Here's how the part is built. I have some questions about the finished solid (model axes, mm). A direction names the side the tool comes from. Round coordinates to 2 decimals unless told otherwise and drop trailing zeros. Write each loop counter-clockwise with the first axis right and the second up, starting at its lowest first coordinate (ties: lowest second). Pieces come first, ordered by that corner, then holes. Notation, with made-up numbers: (-15.5, -12) -> (-9.5, -12) arc R23 ccw to (-9.5, 15) -> close; hole circle Ø10 at (80, 14.25). An arc over 180 degrees is marked (long way). Put each result on its own line as item: value. Start each with the question number.
1. For pin 1 (5 mm diameter, centred on y = 6.5, z = 2199, fed in from +X); pin 2 (10 mm diameter, centred on y = 32, z = 901.5, fed in from -X); pin 3 (5 mm diameter, centred on x = 27, y = -12, fed in from -Z), each with a flat end and sliding along its axis, tell me the tip position at first contact or that it passes through.
2. I need wall thicknesses on probe 1 along Y at (x, z) = (33.5, 731); probe 2 along Y at (x, z) = (-6.5, 903.5); probe 3 along X at (y, z) = (20, 2338). Which ranges of each line are inside material? Lowest first, please. Write a range as from..to.
3. Which directions (+Z, -Z, +X, -X, +Y, -Y) give clear straight access to the entire face, cutting with the end or side of a thin tool? Please do faces 1 (the face through (-62.264, -36.012, 1355.242)), 2 (the face through (67, -37, 2743.2)), 3 (the face through (62.264, 36.012, 1355.242)).
4. Suppose I cut it at A-A (z = 2237.5). Please give me the cut outline in (x, y), then the cut area to 3 significant figures.
```python
from build123d import *

# Parameters (mm, degrees)
F1_DEPTH     = 2540
F3_DEPTH     = 203.2
F4_R         = 76.1921609871
F5_DEPTH     = 101.6
F6_SIZE2     = 203.2
F6_SIZE      = 71.882
F7_T1_DEPTH  = 494.4083201135
F7_T3_DEPTH  = 494.4083201135
F7_T5_DEPTH  = 494.4083201135
F7_T7_DEPTH  = 494.4083201135
F7_T9_DEPTH  = 494.4083201135
F7_T11_DEPTH = 494.4083201135


# Not quite as in the source:
# - a fillet or chamfer that OpenCascade refuses, or shapes differently, is made with other operations: its cross-section is extruded or revolved along the edge and cut away or added


with BuildPart() as f1:
    # F0 (on Top) → F1 (new body)
    with BuildSketch(Plane.XY):
        Polygon((42.1619373396, -71.5559341018), (83.0502253935, 0.735341758), (40.8882880539, 72.2912758598), (-42.1619373396, 71.5559341018), (-83.0502253935, -0.735341758), (-40.8882880539, -72.2912758598), align=None)
    extrude(amount=F1_DEPTH)

    # F2 (on face) → F3 (join)
    with BuildSketch(Plane.XY.offset(2540)):
        with BuildLine():
            ThreePointArc((-40.8882880539, -72.2912758598), (0.735341758, -83.0502253935), (42.1619373396, -71.5559341018))
            Line((42.1619373396, -71.5559341018), (-40.8882880539, -72.2912758598))
        make_face()
        with BuildLine():
            ThreePointArc((-83.0502253935, -0.735341758), (-71.5559341018, -42.1619373396), (-40.8882880539, -72.2912758598))
            Line((-40.8882880539, -72.2912758598), (-83.0502253935, -0.735341758))
        make_face()
        with BuildLine():
            Line((-83.0502253935, -0.735341758), (-42.1619373396, 71.5559341018))
            ThreePointArc((-42.1619373396, 71.5559341018), (-72.2912758598, 40.8882880539), (-83.0502253935, -0.735341758))
        make_face()
        Polygon((42.1619373396, -71.5559341018), (83.0502253935, 0.735341758), (40.8882880539, 72.2912758598), (-42.1619373396, 71.5559341018), (-83.0502253935, -0.735341758), (-40.8882880539, -72.2912758598), align=None)
        with BuildLine():
            ThreePointArc((42.1619373396, -71.5559341018), (72.1095566371, -41.2079180135), (83.0534807543, 0))
            ThreePointArc((83.0534807543, 0), (83.0526669101, 0.3676744818), (83.0502253935, 0.735341758))
            Line((83.0502253935, 0.735341758), (42.1619373396, -71.5559341018))
        make_face()
        with BuildLine():
            Line((40.8882880539, 72.2912758598), (83.0502253935, 0.735341758))
            ThreePointArc((83.0502253935, 0.735341758), (71.5559341018, 42.1619373396), (40.8882880539, 72.2912758598))
        make_face()
        with BuildLine():
            Line((-42.1619373396, 71.5559341018), (40.8882880539, 72.2912758598))
            ThreePointArc((40.8882880539, 72.2912758598), (-0.735341758, 83.0502253935), (-42.1619373396, 71.5559341018))
        make_face()
    extrude(amount=F3_DEPTH)

    # F4 (on face) → F5 (join)
    with BuildSketch(Plane.XY.offset(2743.2)):
        Circle(F4_R)
    extrude(amount=F5_DEPTH)

    # F6
    f6_edges = [f1.edges().sort_by_distance(p)[0] for p in [
        (62.606081, -35.410296, 0),
        (61.969257, 36.513309, 0),
        (-0.636825, 71.923605, 0),
        (-62.606081, 35.410296, 0),
        (-61.969257, -36.513309, 0),
        (0.636825, -71.923605, 0),
    ]]
    f6_side = f1.faces().sort_by_distance((0, 0, 0))[0]
    chamfer(f6_edges, length=F6_SIZE, length2=F6_SIZE2, reference=f6_side)

    # F7: fillet of radius 76.2 on 6 edges, made by hand

    # F7_s2 → F7_t1 (cut)
    with BuildSketch(Plane(origin=(-18.9514614698, -33.5065465998, -94.2401135792), x_dir=(-0.8704183762, 0.4923127566, 0), z_dir=(0.1861654151, 0.329144017, 0.9257465389))):
        with BuildLine():
            ThreePointArc((-35.9188045712, 19.1503954496), (0, 10.1536652969), (35.9188045712, 19.1503954496))
            Line((35.9188045712, 19.1503954496), (0, -0.0474877004))
            Line((0, -0.0474877004), (-35.9188045712, 19.1503954496))
        make_face()
    extrude(amount=F7_T1_DEPTH, mode=Mode.SUBTRACT)

    # F7_s4 → F7_t3 (cut)
    with BuildSketch(Plane(origin=(19.5417898136, -33.1657203716, -94.2401135792), x_dir=(-0.8615645419, -0.5076480475, 0), z_dir=(-0.1919643727, 0.3257959873, 0.9257465389))):
        with BuildLine():
            ThreePointArc((-35.9188045712, 19.1503954496), (0, 10.1536652969), (35.9188045712, 19.1503954496))
            Line((35.9188045712, 19.1503954496), (0, -0.0474877004))
            Line((0, -0.0474877004), (-35.9188045712, 19.1503954496))
        make_face()
    extrude(amount=F7_T3_DEPTH, mode=Mode.SUBTRACT)

    # F7_s6 → F7_t5 (cut)
    with BuildSketch(Plane(origin=(38.4932512834, 0.3408262282, -94.2401135792), x_dir=(0.0088538343, -0.999960804, 0), z_dir=(-0.3781297878, -0.0033480297, 0.9257465389))):
        with BuildLine():
            ThreePointArc((35.9188045712, 19.1503954496), (0, 10.1536652969), (-35.9188045712, 19.1503954496))
            Line((-35.9188045712, 19.1503954496), (0, -0.0474877004))
            Line((0, -0.0474877004), (35.9188045712, 19.1503954496))
        make_face()
    extrude(amount=F7_T5_DEPTH, mode=Mode.SUBTRACT)

    # F7_s8 → F7_t7 (cut)
    with BuildSketch(Plane(origin=(18.9514614698, 33.5065465998, -94.2401135792), x_dir=(0.8704183762, -0.4923127566, 0), z_dir=(-0.1861654151, -0.329144017, 0.9257465389))):
        with BuildLine():
            ThreePointArc((35.9188045712, 19.1503954496), (0, 10.1536652969), (-35.9188045712, 19.1503954496))
            Line((-35.9188045712, 19.1503954496), (0, -0.0474877004))
            Line((0, -0.0474877004), (35.9188045712, 19.1503954496))
        make_face()
    extrude(amount=F7_T7_DEPTH, mode=Mode.SUBTRACT)

    # F7_s10 → F7_t9 (cut)
    with BuildSketch(Plane(origin=(-19.5417898136, 33.1657203716, -94.2401135792), x_dir=(0.8615645419, 0.5076480475, 0), z_dir=(0.1919643727, -0.3257959873, 0.9257465389))):
        with BuildLine():
            ThreePointArc((35.9188045712, 19.1503954496), (0, 10.1536652969), (-35.9188045712, 19.1503954496))
            Line((-35.9188045712, 19.1503954496), (0, -0.0474877004))
            Line((0, -0.0474877004), (35.9188045712, 19.1503954496))
        make_face()
    extrude(amount=F7_T9_DEPTH, mode=Mode.SUBTRACT)

    # F7_s12 → F7_t11 (cut)
    with BuildSketch(Plane(origin=(-38.4932512834, -0.3408262282, -94.2401135792), x_dir=(-0.0088538343, 0.999960804, 0), z_dir=(0.3781297878, 0.0033480297, 0.9257465389))):
        with BuildLine():
            ThreePointArc((-35.9188045712, 19.1503954496), (0, 10.1536652969), (35.9188045712, 19.1503954496))
            Line((35.9188045712, 19.1503954496), (0, -0.0474877004))
            Line((0, -0.0474877004), (-35.9188045712, 19.1503954496))
        make_face()
    extrude(amount=F7_T11_DEPTH, mode=Mode.SUBTRACT)


solid = f1.part
```
Verdict:
1. pin 1: stops at x = 81.13
1. pin 2: stops at x = -67.36
1. pin 3: stops at z = 89.09
2. probe 1: y = -71.63..72.23
2. probe 2: y = -71.99..71.87
2. probe 3: x = -71.32..71.7
3. face 1: -Z, -X, -Y
3. face 2: +Z
3. face 3: -Z, +X, +Y
4. outline: (-83.05, -0.74) -> (-40.89, -72.29) -> (42.16, -71.56) -> (83.05, 0.74) -> (40.89, 72.29) -> (-42.16, 71.56) -> close
4. area: 17,900 mm^2
